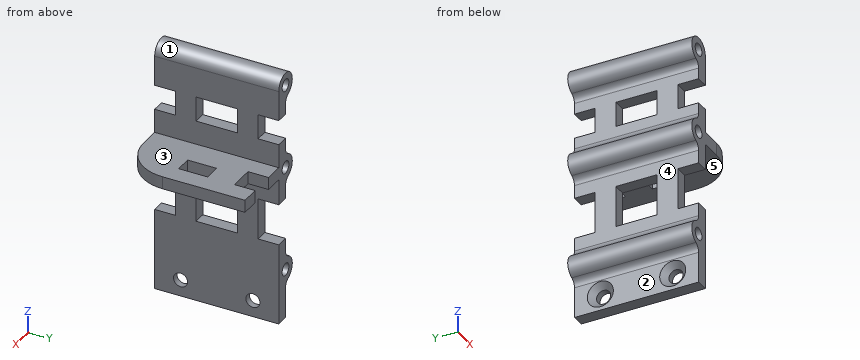
from build123d import *

# Parameters (mm, degrees)
BOSS_EXTRUDE1_DEPTH                                 = 30
CSK_FOR_M3_COUNTERSUNK_FLAT_HEAD_SCREW1_D           = 3.4
CSK_FOR_M3_COUNTERSUNK_FLAT_HEAD_SCREW1_CSINK_D     = 6.3
CSK_FOR_M3_COUNTERSUNK_FLAT_HEAD_SCREW1_CSINK_ANGLE = 90
SKETCH4_R                                           = 3
BOSS_EXTRUDE2_DEPTH                                 = 30
SKETCH5_R                                           = 1.5
CUT_EXTRUDE1_DEPTH                                  = 71.320693967
CUT_EXTRUDE2_REACH                                  = 52.2
SKETCH7_W                                           = 4
SKETCH7_H                                           = 7
CUT_EXTRUDE3_REACH                                  = 72.321
SKETCH10_W                                          = 10
SKETCH10_H                                          = 5
SKETCH10_W_2                                        = 6
SKETCH10_H_2                                        = 10
CUT_EXTRUDE4_REACH                                  = 54.393
SKETCH11_W                                          = 6
SKETCH11_H                                          = 5
FILLET1_R                                           = 2
FILLET2_R                                           = 10


with BuildPart() as part:
    # Sketch1 → Boss-Extrude1 (new body)
    with BuildSketch(Plane(origin=(0, 0, 0), x_dir=(1, 0, 0), z_dir=(0, 1, 0))):
        Polygon((0, -58), (0, 0), (3, 0), (3, -36), (18, -36), (18, -39), (3, -39), (3, -58), align=None)
    extrude(amount=BOSS_EXTRUDE1_DEPTH)

    # CSK for M3 Countersunk Flat Head Screw1 (through all)
    with Locations(Plane.ZY):
        with Locations((4, 23.75), (4, 6.25)):
            CounterSinkHole(CSK_FOR_M3_COUNTERSUNK_FLAT_HEAD_SCREW1_D / 2, CSK_FOR_M3_COUNTERSUNK_FLAT_HEAD_SCREW1_CSINK_D / 2, counter_sink_angle=CSK_FOR_M3_COUNTERSUNK_FLAT_HEAD_SCREW1_CSINK_ANGLE)

    # Sketch4 → Boss-Extrude2 (add)
    with BuildSketch(Plane(origin=(0, 0, 0), x_dir=(1, 0, 0), z_dir=(0, 1, 0))):
        with Locations((0, -12)):
            Circle(SKETCH4_R)
        with Locations((0, -37.5)):
            Circle(SKETCH4_R)
        with Locations((0, -58)):
            Circle(SKETCH4_R)
    extrude(amount=BOSS_EXTRUDE2_DEPTH)

    # Sketch5 → Cut-Extrude1 (cut, through all)
    with BuildSketch(Plane(origin=(0, 30, 0), x_dir=(1, 0, 0), z_dir=(0, 1, 0))):
        with Locations(Location((0, -12, 0), (0, 0, 270))):
            Circle(SKETCH5_R)
        with Locations(Location((0, -37.5, 0), (0, 0, 270))):
            Circle(SKETCH5_R)
        with Locations(Location((0, -58, 0), (0, 0, 270))):
            Circle(SKETCH5_R)
    extrude(amount=-CUT_EXTRUDE1_DEPTH, mode=Mode.SUBTRACT)

    # Sketch7 → Cut-Extrude2 (cut, up to next)
    with BuildSketch(Plane(origin=(0, 0, 36), x_dir=(-1, 0, 0), z_dir=(0, 0, -1)), mode=Mode.PRIVATE) as cut_extrude2_sk1:
        with Locations((-11.5, 15)):
            Rectangle(SKETCH7_W, SKETCH7_H)
    cut_extrude2_tool1 = extrude(cut_extrude2_sk1.sketch, amount=-CUT_EXTRUDE2_REACH, mode=Mode.PRIVATE) & part.part
    add(cut_extrude2_tool1.solids().sort_by_distance((11.5, 15, 36))[0], mode=Mode.SUBTRACT)

    # Sketch10 → Cut-Extrude3 (cut, up to next)
    with BuildSketch(Plane.ZY, mode=Mode.PRIVATE) as cut_extrude3_sk1:
        with Locations((24.75, 27.5)):
            Rectangle(SKETCH10_W, SKETCH10_H)
    cut_extrude3_tool1 = extrude(cut_extrude3_sk1.sketch, amount=-CUT_EXTRUDE3_REACH, mode=Mode.PRIVATE) & part.part
    # Sketch10 → Cut-Extrude3 (cut, up to next)
    with BuildSketch(Plane.ZY, mode=Mode.PRIVATE) as cut_extrude3_sk2:
        with Locations((47.75, 27.5)):
            Rectangle(SKETCH10_W_2, SKETCH10_H)
    cut_extrude3_tool2 = extrude(cut_extrude3_sk2.sketch, amount=-CUT_EXTRUDE3_REACH, mode=Mode.PRIVATE) & part.part
    # Sketch10 → Cut-Extrude3 (cut, up to next)
    with BuildSketch(Plane.ZY, mode=Mode.PRIVATE) as cut_extrude3_sk3:
        with Locations((24.75, 2.5)):
            Rectangle(SKETCH10_W, SKETCH10_H)
    cut_extrude3_tool3 = extrude(cut_extrude3_sk3.sketch, amount=-CUT_EXTRUDE3_REACH, mode=Mode.PRIVATE) & part.part
    # Sketch10 → Cut-Extrude3 (cut, up to next)
    with BuildSketch(Plane.ZY, mode=Mode.PRIVATE) as cut_extrude3_sk4:
        with Locations((47.75, 2.5)):
            Rectangle(SKETCH10_W_2, SKETCH10_H)
    cut_extrude3_tool4 = extrude(cut_extrude3_sk4.sketch, amount=-CUT_EXTRUDE3_REACH, mode=Mode.PRIVATE) & part.part
    # Sketch10 → Cut-Extrude3 (cut, up to next)
    with BuildSketch(Plane.ZY, mode=Mode.PRIVATE) as cut_extrude3_sk5:
        with Locations((24.75, 15)):
            Rectangle(SKETCH10_W, SKETCH10_H_2)
    cut_extrude3_tool5 = extrude(cut_extrude3_sk5.sketch, amount=-CUT_EXTRUDE3_REACH, mode=Mode.PRIVATE) & part.part
    # Sketch10 → Cut-Extrude3 (cut, up to next)
    with BuildSketch(Plane.ZY, mode=Mode.PRIVATE) as cut_extrude3_sk6:
        with Locations((47.75, 15)):
            Rectangle(SKETCH10_W_2, SKETCH10_H_2)
    cut_extrude3_tool6 = extrude(cut_extrude3_sk6.sketch, amount=-CUT_EXTRUDE3_REACH, mode=Mode.PRIVATE) & part.part
    add(cut_extrude3_tool1.solids().sort_by_distance((0, 27.5, 24.75))[0], mode=Mode.SUBTRACT)
    add(cut_extrude3_tool2.solids().sort_by_distance((0, 27.5, 47.75))[0], mode=Mode.SUBTRACT)
    add(cut_extrude3_tool3.solids().sort_by_distance((0, 2.5, 24.75))[0], mode=Mode.SUBTRACT)
    add(cut_extrude3_tool4.solids().sort_by_distance((0, 2.5, 47.75))[0], mode=Mode.SUBTRACT)
    add(cut_extrude3_tool5.solids().sort_by_distance((0, 15, 24.75))[0], mode=Mode.SUBTRACT)
    add(cut_extrude3_tool6.solids().sort_by_distance((0, 15, 47.75))[0], mode=Mode.SUBTRACT)

    # Sketch11 → Cut-Extrude4 (cut, up to next)
    with BuildSketch(Plane.XY.offset(39), mode=Mode.PRIVATE) as cut_extrude4_sk1:
        with Locations((10.5, 27.5)):
            Rectangle(SKETCH11_W, SKETCH11_H)
    cut_extrude4_tool1 = extrude(cut_extrude4_sk1.sketch, amount=-CUT_EXTRUDE4_REACH, mode=Mode.PRIVATE) & part.part
    add(cut_extrude4_tool1.solids().sort_by_distance((10.5, 27.5, 39))[0], mode=Mode.SUBTRACT)

    # Fillet1
    fillet1_edges = [part.edges().sort_by_distance(p)[0] for p in [
        (0, 15, 15),
        (0, 15, 9),
        (0, 15, 40.5),
        (0, 15, 34.5),
        (0, 15, 55),
    ]]
    fillet(fillet1_edges, radius=FILLET1_R)

    # Fillet2
    fillet2_edges = [part.edges().sort_by_distance(p)[0] for p in [
        (18, 0, 37.5),
    ]]
    fillet(fillet2_edges, radius=FILLET2_R)


solid = part.part
The model under review builds one solid part; all positions refer to its coordinate system, in mm. Face numbers are marked on the shaded views. A direction names the side the tool comes from. Give positions to 0.01 mm unless a question says otherwise; leave off trailing zeros. Write each loop counter-clockwise with the first axis right and the second up, starting at its lowest first coordinate (ties: lowest second). Pieces come first, ordered by that corner, then holes.
1. Add section A-A, the plane z = 37.5. Write out the cut boundary in (x, y), plus the area to 3 significant figures.
2. Add section C-C, the plane z = 12. Write out the cut boundary in (x, y), plus the area to 3 significant figures.
3. Wall thickness on L1, parallel to Y at x = 2.2, z = 4; L2, parallel to X at y = 11, z = 58; L3, parallel to Z at x = -1, y = 15: over which ranges is each line inside the solid? List them lowest first.
4. Add section D-D, the plane y = 6.25. Write out the cut boundary in (x, z), plus the area to 3 significant figures.
5. Add section B-B, the plane y = 15.75. Count the separate pieces of the cut face and the enclosed holes in it, plus the area to 3 significant figures.
6. For P1, Ø2.5, axis at x = 11, z = 37.5, coming from the +Y side; P2, Ø1.5, axis at x = 3, y = 3.5, coming from the +Z side; P3, Ø2.5, axis at x = 12.5, z = 37, coming from the -Y side; P4, Ø2.5, axis at x = 0, z = 12, coming from the +Y side, all flat-tipped, find the tip position at first contact; note any pin that passes through.
7. Tool access review of the marked faces 1, 2, 3, 4 and 5: name each direction out of +Z, -Z, +X, -X, +Y, -Y from which nothing blocks a thin tool from reaching the whole face with its end or side.
Worked answers:
1. outline: (-3, 0) - (-1.5, 0) - (-1.5, 30) - (-3, 30) - close; (1.5, 0) - (8, 0) arc R10 ccw to (18, 10) - (18, 30) - (13.5, 30) - (13.5, 25) - (7.5, 25) - (7.5, 30) - (1.5, 30) - close; hole (9.5, 11.5) - (13.5, 11.5) - (13.5, 18.5) - (9.5, 18.5) - close
1. area: 461 mm2
2. outline: (-3, 0) - (-1.5, 0) - (-1.5, 30) - (-3, 30) - close; (1.5, 0) - (3, 0) - (3, 30) - (1.5, 30) - close
2. area: 90.0 mm2
3. L1: y = 0 to 4.55, 7.95 to 22.05, 25.45 to 30
3. L2: x = -3 to -1.5, 1.5 to 3
3. L3: z = 9.15 to 10.88, 13.12 to 14.85, 34.65 to 36.38, 38.62 to 40.35, 55.15 to 56.88, 59.12 to 60.83
4. outline: (-1.2, 9.25) arc R2 cw to (0, 7.42) - (0, 7.15) - (1.45, 5.7) - (3, 5.7) - (3, 36) - (17.27, 36) - (17.27, 39) - (3, 39) - (3, 58) arc R3 ccw (long way) to (-1.2, 55.25) arc R2 cw to (0, 53.42) - (0, 42.08) arc R2 cw to (-1.2, 40.25) arc R3 ccw to (-1.2, 34.75) arc R2 cw to (0, 32.92) - (0, 16.58) arc R2 cw to (-1.2, 14.75) arc R3 ccw to start; (0, 0) - (3, 0) - (3, 2.3) - (1.45, 2.3) - (0, 0.85) - close; hole circle Ø3 at (0, 12); hole circle Ø3 at (0, 37.5); hole circle Ø3 at (0, 58)
4. area: 235 mm2
5. separate pieces: 4
5. enclosed holes: 3
5. area: 189 mm2
6. P1: stops at y = 25
6. P2: stops at z = 59.98
6. P3: stops at y = 0.54
6. P4: passes through
7. face 1: +Y, -Y
7. face 2: -Z, -X, +Y, -Y
7. face 3: +Z, +X, +Y, -Y
7. face 4: -X, +Y, -Y
7. face 5: -Z, +X, +Y, -Y
